The model under review builds one solid part; all positions refer to its coordinate system, in mm. Face numbers are marked on the shaded views. Coordinates: 2 decimals unless noted, no trailing zeros. Write each loop counter-clockwise with the first axis right and the second up, starting at its lowest first coordinate (ties: lowest second). Pieces come first, ordered by that corner, then holes. Notation, with made-up numbers: M -9.5,75 L 21.5,75 A18 ccw 21.5,93 Z; hole C 77,-8 d7. An arc over 180 degrees is marked long. Answer as a JSON object with one key per item and string values.
```python
from build123d import *

# Parameters (mm, degrees)
SKETCH3_R   = 63.5
SKETCH3_R_2 = 51.1302


with BuildPart() as part:
    # Sketch1 → Revolve1 (revolve)
    with BuildSketch(Plane.XY):
        Polygon((-10.664054144, -100.466615354), (25.256970341, -64.54559087), (20.686019975, -59.974640505), (-14.992537594, -96.138131904), align=None)
    revolve(axis=Axis((-55.565334749, -55.565334749, 0), (0.707106781, 0.707106781, 0)))



with BuildPart() as body_2:
    # Sketch2 → Revolve2 (revolve)
    with BuildSketch(Plane.XY):
        Polygon((57.3786, 78.58125), (57.0357, 27.78125), (63.5, 27.78125), (63.5, 78.58125), align=None)
    revolve(axis=Axis((0, 0, 0), (0, 1, 0)))


with BuildPart() as part_1:
    add(part.part)

    add(body_2.part)  # Sweep1 merges body 2
    # Sweep1: sweep along a path in Sketch4
    with BuildLine(Plane.XY) as sweep1_path:
        ThreePointArc((-19.644310265, -19.644310265), (-5.105389899, 2.114721737), (0, 27.78125))
    # Sketch3 → Sweep1 (sweep)
    with BuildSketch(Plane(origin=(-19.644310265, -19.644310265, 0), x_dir=(0, 0, -1), z_dir=(0.707106781, 0.707106781, 0))):
        Circle(SKETCH3_R)
        Circle(SKETCH3_R_2, mode=Mode.SUBTRACT)
    sweep(path=sweep1_path.line)


solid = part_1.part
```
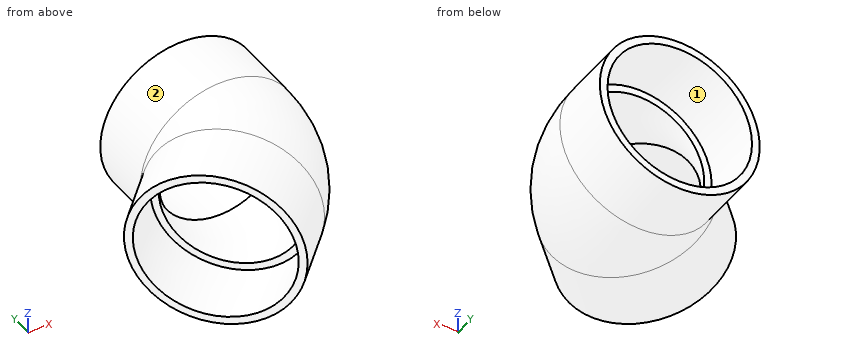
(1) Wall thickness on line 1 along Z through (x, y) = (-10.5, -7.5); line 2 along X through (y, z) = (43, -5); line 3 along Z through (x, y) = (-2.5, -44): over which ranges is each line inside the solid? List them lowest first. Write a range as from..to.
Results list:
{"line 1": "-63.5..-51.13, 51.13..63.5", "line 2": "-63.3..-56.92, 56.92..63.3", "line 3": "-56.31..-48.95, 48.95..56.31"}
(2) Add section A-A on y = 38. Give the boundary of the cut face in (x, z), and give its area (3 significant figures).
Results list:
{"outline": "C 0,0 d127; hole C 0,0 d114.21", "area": "2,420 mm²"}
(3) Draft analysis for pull direction X (two halves, no side actions). For the marked faces 1 and 2, state which applies: released by +X, released by -X, zero draft, split by the parting line, or undercut.
Results list:
{"face 1": "undercut", "face 2": "split by the parting line"}
(4) For pin 1 Ø1.5 at (x, y) = (3.5, -0.5) entering from -Z; pin 2 Ø2 at (y, z) = (38, -29) entering from -X; pin 3 Ø10 at (y, z) = (-2, -25.5) entering from -X, all flat-tipped, find the tip position at first contact; note any pin that passes through.
Results list:
{"pin 1": "z = -62.97", "pin 2": "x = -56.99", "pin 3": "x = -90.04"}
